Verification items for the finished model (mm, model axes). A direction names the side the tool comes from. Round coordinates to 2 decimals unless told otherwise and drop trailing zeros. Write each loop counter-clockwise with the first axis right and the second up, starting at its lowest first coordinate (ties: lowest second). Pieces come first, ordered by that corner, then holes. Notation, with made-up numbers: (77, 13.5) -> (134, 13.5) arc R15 ccw to (134, 18.5) -> close; hole circle Ø10 at (-39.5, 34). An arc over 180 degrees is marked (long way). Answer as a JSON object with one key per item and string values. Group by question number.
(1) Gauge pin test, flat ends, axial feed: pin 1 Ø4 at (y, z) = (-19, 3.5) entering from +X; pin 2 Ø2 at (x, y) = (-10.5, -21) entering from +Z; pin 3 Ø1 at (x, z) = (10.5, 8) entering from +Y; pin 4 Ø3 at (x, y) = (11.39, -22.84) entering from -Z. Record the tip position at first contact, or that the pin passes through.
(2) Sectioned sample at C-C on z = 1.25. Record the cut outline in (x, y) (3 decimals).
(3) Draft check along Z on faces 4 (the face through (0, -34, 12.7)), 5 (the face through (-23.89, -24.217, 5.857)), 6 (the face through (0, -25, 0)), 7 (the face through (13.15, -23.57, 1.29)). Enter one of: released by +Z, released by -Z, zero draft, split by the parting line, or undercut.
(4) Scan lines: L1, parallel to Z at x = 18, y = -26.25; L2, parallel to X at y = -26, z = 11.25; L3, parallel to X at y = -29.5, z = 11.25. Record each from-to range of solid material in increasing order. Write a range as from..to.
(5) Set-up check for faces 1 (the face through (0, -25, 2.54)), 2 (the face through (-28.11, -19.683, 3.439)), 3 (the face through (-18.19, -17.73, 1.25)): record each of +Z, -Z, +X, -X, +Y, -Y from which the full face is reachable in a straight line by a thin tool's end or side.
(6) Sectioned sample at A-A on x = 10.5. Record the cut outline in (y, z).
(7) Sectioned sample at B-B on y = -33.25. Record the cut outline in (x, z), and give its area (3 significant figures).
(8) Sectioned sample at D-D on x = 4.5. Record the cut outline in (y, z).
Autodesk Inventor part; units mm, degrees
ref_plane "Work Plane2" through (25.1447, -25.1447, 0) normal (0.7071068, -0.7071068, 0) x (0.7071068, 0.7071068, 0)
ref_plane "Work Plane4" through (-25.1447, -25.1447, 0) normal (0.7071068, 0.7071068, 0) x (-0.7071068, 0.7071068, 0)
ref_plane "XZ Plane" through (0, 0, 0) normal (0, 1, 0) x (-1, 0, 0)
sketch "Sketch1" plane through (0, 0, 0) normal (0, 0, 1) x (1, 0, 0)
  arc A0 (-20.8065, -14.5688) -> (20.8065, -14.5688) centre (0, 0) ccw
  arc A1 (-29.129, -20.3964) -> (29.129, -20.3964) centre (0, 0) ccw
  line L0 (-29.129, -20.3964) -> (-20.8065, -14.5688)
  line L1 (29.129, -20.3964) -> (20.8065, -14.5688)
  line L2 (-20.8065, -14.5688) -> (20.8065, -14.5688) construction
  dimension "d0" = 50.8
  dimension "d2" = 71.12
  dimension "d3" = 110
extrude "Extrusion1" add sketch "Sketch1" along normal blind 2.54
sketch "Sketch2" plane through (0, 0, 2.54) normal (0, 0, 1) x (1, 0, 0)
  arc A0 (-20.8065, -14.5688) -> (20.8065, -14.5688) centre (0, 0) ccw
  line L0 (-14.5688, -20.8065) -> (-13.112, -18.7258)
  line L1 (14.5688, -20.8065) -> (13.112, -18.7258)
  arc A1 (-13.112, -18.7258) -> (13.112, -18.7258) centre (0, 0) ccw
  line L2 (-14.5688, -20.8065) -> (14.5688, -20.8065) construction
  dimension "d6" = 2.54
  dimension "d13" = 70
extrude "Extrusion2" add sketch "Sketch2" against normal blind 2.54
sketch "Sketch3" plane through (0, 0, 2.54) normal (0, 0, 1) x (1, 0, 0)
  circle A0 centre (-11.3901, -22.845) radius 1.905
  circle A1 centre (11.3901, -22.845) radius 1.905
  line L0 (-11.3901, -22.845) -> (11.3901, -22.845) construction
  point P0 (0, 0)
  point P1 (0, -22.845)
  dimension "d9" = 3.81
  dimension "d10" = 3.81
  dimension "d11" = 25.527
  dimension "d12" = 26.5
extrude "Extrusion3" cut sketch "Sketch3" against normal through all
sketch "Sketch4" plane through (0, 0, 2.54) normal (0, 0, 1) x (1, 0, 0)
  circle A0 centre (-11.3901, -22.845) radius 1.905
  circle A1 centre (11.3901, -22.845) radius 1.905
  arc A2 (-29.129, -20.3964) -> (29.129, -20.3964) centre (0, 0) ccw
  line L0 (29.129, -20.3964) -> (20.8065, -14.5688)
  arc A3 (14.5688, -20.8065) -> (20.8065, -14.5688) centre (0, 0) ccw
  line L1 (14.5688, -20.8065) -> (13.112, -18.7258)
  arc A4 (-13.112, -18.7258) -> (13.112, -18.7258) centre (0, 0) ccw
  line L2 (-13.112, -18.7258) -> (-14.5688, -20.8065)
  arc A5 (-20.8065, -14.5688) -> (-14.5688, -20.8065) centre (0, 0) ccw
  line L3 (-20.8065, -14.5688) -> (-29.129, -20.3964)
  line L4 (-20.8065, -14.5688) -> (-29.129, -20.3964)
  line L5 (29.129, -20.3964) -> (20.8065, -14.5688)
  arc A6 (-27.6726, -19.3766) -> (27.6726, -19.3766) centre (0, 0) ccw
  dimension "d17" = 67.564
extrude "Extrusion4" add sketch "Sketch4" along normal blind 10.16 contours L3 A6 L0 A2
ref_plane "Work Plane2" through (25.1447, -25.1447, 0) normal (0.7071068, -0.7071068, 0) x (0.7071068, 0.7071068, 0)
ref_plane "Work Plane1" through (0, 0, 2.54) normal (0.7071068, -0.7071068, 0) x (0, 0, -1)
ref_plane "Work Plane4" through (-25.1447, -25.1447, 0) normal (0.7071068, 0.7071068, 0) x (-0.7071068, 0.7071068, 0)
ref_plane "Work Plane3" through (0, 0, 2.54) normal (0.7071068, 0.7071068, 0) x (0, 0, -1)
sketch "Sketch5" plane through (-25.1447, -25.1447, 0) normal (0.7071068, 0.7071068, 0) x (-0.7071068, 0.7071068, 0)
  circle A0 centre (0, 7.62) radius 1.778
  line L0 (5.8662, 2.54) -> (5.8662, 12.7)
  point P0 (0, 0)
  point P1 (6.1749, 4.826)
  point P2 (5.8662, 7.62)
  dimension "d22" = 3.556
extrude "Extrusion5" cut sketch "Sketch5" along normal blind 7.112
sketch "Sketch6" plane through (25.1447, -25.1447, 0) normal (0.7071068, -0.7071068, 0) x (0.7071068, 0.7071068, 0)
  circle A0 centre (0, 7.62) radius 1.778
  line L0 (5.8662, 2.54) -> (5.8662, 12.7)
  point P0 (0, 0)
  point P1 (6.1749, 4.826)
  point P2 (5.8662, 7.62)
  dimension "d25" = 3.556
extrude "Extrusion6" cut sketch "Sketch6" against normal blind 7.112
fillet "Fillet1" radius 3.175 6 edges at (-20.8065, -14.5688, 1.27) (-14.5688, -20.8065, 1.27) (-13.112, -18.7258, 1.27) (13.112, -18.7258, 1.27) (14.5688, -20.8065, 1.27) (20.8065, -14.5688, 1.27)
chamfer "Chamfer1" distance 1.27 angle 45 2 edges at (-23.856, -26.3705, 7.6201) (23.856, -26.3705, 7.6201)
properties part number "BearingMountBrace" material "ABS Plastic"
Computed values:
{
 "1": {"pin 1": "x = 29.13", "pin 2": "z = 2.54", "pin 3": "y = -31.94", "pin 4": "through"},
 "2": {"outline": "(-29.129, -20.396) arc R35.56 ccw to (29.129, -20.396) -> (23.262, -16.288) arc R3.175 ccw to (19.059, -16.79) arc R25.4 cw to (17.295, -18.602) arc R3.175 cw to (14.23, -19.321) arc R3.175 ccw to (11.702, -19.638) arc R22.86 cw to (-11.702, -19.638) arc R3.175 ccw to (-14.23, -19.321) arc R3.175 cw to (-17.295, -18.602) arc R25.4 cw to (-19.059, -16.79) arc R3.175 ccw to (-23.262, -16.288) -> close; hole circle Ø3.81 at (-11.39, -22.845); hole circle Ø3.81 at (11.39, -22.845)"},
 "3": {"face 4": "released by +Z", "face 5": "undercut", "face 6": "released by -Z", "face 7": "zero draft"},
 "4": {"L1": "0..2.54", "L2": "-24.26..-21.57, 21.57..24.26", "L3": "-19.86..-16.46, 16.46..19.86"},
 "5": {"face 1": "+Z, +Y", "face 2": "+Z, -Z, -X, +Y", "face 3": "+Z, -Z, +Y"},
 "6": {"outline": "(-33.97, 0) -> (-24.53, 0) -> (-24.53, 2.54) -> (-32.11, 2.54) -> (-32.11, 12.7) -> (-33.97, 12.7) -> close; (-21.16, 0) -> (-20.31, 0) -> (-20.31, 2.54) -> (-21.16, 2.54) -> close"},
 "7": {"outline": "(-12.61, 0) -> (12.61, 0) -> (12.61, 12.7) -> (5.97, 12.7) -> (5.97, 2.54) -> (-5.97, 2.54) -> (-5.97, 12.7) -> (-12.61, 12.7) -> close", "area": "199 mm2"},
 "8": {"outline": "(-35.27, 0) -> (-22.41, 0) -> (-22.41, 2.54) -> (-33.48, 2.54) -> (-33.48, 12.7) -> (-35.27, 12.7) -> close"}
}
